from build123d import *

# Parameters (mm, degrees)
BOSS_EXTRUDE1_DEPTH   = 116
SKETCH5_R             = 16
CUT_EXTRUDE1_DEPTH    = 20
CUT_EXTRUDE2_REACH    = 6.51
SKETCH6_R             = 10
CUT_EXTRUDE4_REACH    = 17
SKETCH8_R             = 45
CUT_EXTRUDE5_DEPTH    = 106
FILLET3_R             = 25
SKETCH21_R            = 55
CUT_EXTRUDE7_DEPTH    = 5
M4X0_7_TAPPED_HOLE1_D = 3.3
FILLET4_R             = 0.8
CHAMFER1_SIZE         = 10
SKETCH25_W            = 64.356
SKETCH25_H            = 48.356
BOSS_EXTRUDE2_DEPTH   = 116
CUT_EXTRUDE8_DEPTH    = 106
FILLET6_R             = 10
FILLET7_R             = 10
FILLET8_R             = 10


with BuildPart() as part:
    # Sketch1 → Boss-Extrude1 (new body)
    with BuildSketch(Plane.XY):
        Polygon((0, 0), (-106, 0), (-121, 0), (-121, 155), (-106, 155), (-106, 16), (-24.51, 16), (-24.51, 107), (0, 107), align=None)
    extrude(amount=-BOSS_EXTRUDE1_DEPTH)

    # Sketch5 → Cut-Extrude1 (cut)
    with BuildSketch(Plane.ZY.offset(24.51)):
        with Locations((-58, 86)):
            Circle(SKETCH5_R)
    extrude(amount=-CUT_EXTRUDE1_DEPTH, mode=Mode.SUBTRACT)

    # Sketch6 → Cut-Extrude2 (cut, up to next)
    with BuildSketch(Plane.ZY.offset(4.51), mode=Mode.PRIVATE) as cut_extrude2_sk1:
        with Locations((-58, 86)):
            Circle(SKETCH6_R)
    cut_extrude2_tool1 = extrude(cut_extrude2_sk1.sketch, amount=-CUT_EXTRUDE2_REACH, mode=Mode.PRIVATE) & part.part
    add(cut_extrude2_tool1.solids().sort_by_distance((-4.51, 86, -58))[0], mode=Mode.SUBTRACT)

    # Sketch8 → Cut-Extrude4 (cut, up to next)
    with BuildSketch(Plane(origin=(-106, 0, 0), x_dir=(0, 0, -1), z_dir=(1, 0, 0)), mode=Mode.PRIVATE) as cut_extrude4_sk1:
        with Locations((58, 86)):
            Circle(SKETCH8_R)
    cut_extrude4_tool1 = extrude(cut_extrude4_sk1.sketch, amount=-CUT_EXTRUDE4_REACH, mode=Mode.PRIVATE) & part.part
    add(cut_extrude4_tool1.solids().sort_by_distance((-106, 86, -58))[0], mode=Mode.SUBTRACT)

    # Sketch10 → Cut-Extrude5 (cut)
    with BuildSketch(Plane(origin=(0, 0, 0), x_dir=(0, 0, -1), z_dir=(1, 0, 0))):
        with BuildLine():
            Line((0, 107), (0, 16))
            Line((0, 16), (23.561161531, 22.820336233))
            ThreePointArc((23.561161531, 22.820336233), (33.987858372, 30.015449722), (38, 42.031621521))
            Line((38, 42.031621521), (38, 87))
            ThreePointArc((38, 87), (43.857864376, 101.142135624), (58, 107))
            Line((58, 107), (0, 107))
        make_face()
        with BuildLine():
            Line((116, 107), (58, 107))
            ThreePointArc((58, 107), (72.142135624, 101.142135624), (78, 87))
            Line((78, 87), (78, 42.031621521))
            ThreePointArc((78, 42.031621521), (82.012141628, 30.015449722), (92.438838469, 22.820336233))
            Line((92.438838469, 22.820336233), (116, 16))
            Line((116, 16), (116, 107))
        make_face()
    extrude(amount=-CUT_EXTRUDE5_DEPTH, mode=Mode.SUBTRACT)

    # Fillet3
    fillet3_edges = [part.edges().sort_by_distance(p)[0] for p in [
        (-113.5, 155, 0),
        (-113.5, 155, -116),
    ]]
    fillet(fillet3_edges, radius=FILLET3_R)

    # Sketch21 → Cut-Extrude7 (cut)
    with BuildSketch(Plane.ZY.offset(121)):
        with Locations((-58, 86)):
            Circle(SKETCH21_R)
    extrude(amount=-CUT_EXTRUDE7_DEPTH, mode=Mode.SUBTRACT)

    # M4x0.7 Tapped Hole1 (through all)
    with Locations(Plane.ZY.offset(116)):
        with Locations((-103.10855484, 107.568919311), (-12.89144516, 107.568919311), (-12.89144516, 64.431080689), (-103.10855484, 64.431080689)):
            Hole(M4X0_7_TAPPED_HOLE1_D / 2)

    # Mirror1: part across plane


with BuildPart() as part_1:
    add(part.part)
    add(part.part.mirror(Plane(origin=(0, 107, -116), x_dir=(0, 0, 1), z_dir=(1, 0, 0))))

    # Fillet4
    fillet4_edges = [part_1.edges().sort_by_distance(p)[0] for p in [
        (4.51, 86, -74),
        (-4.51, 86, -74),
    ]]
    fillet(fillet4_edges, radius=FILLET4_R)

    # Chamfer1
    chamfer1_edges = [part_1.edges().sort_by_distance(p)[0] for p in [
        (-121, 0, -58),
        (121, 0, -58),
    ]]
    chamfer(chamfer1_edges, length=CHAMFER1_SIZE)

    # Sketch25 → Boss-Extrude2 (add)
    with BuildSketch(Plane.XY):
        with Locations((0, -24.178)):
            Rectangle(SKETCH25_W, SKETCH25_H)
    extrude(amount=-BOSS_EXTRUDE2_DEPTH)

    # Sketch27 → Cut-Extrude8 (cut)
    with BuildSketch(Plane(origin=(0, 0, -116), x_dir=(-1, 0, 0), z_dir=(0, 0, -1))):
        with BuildLine():
            Line((-21.05025, -43.356), (21.05025, -43.356))
            ThreePointArc((21.05025, -43.356), (25.383223578, -41.561223578), (27.178, -37.22825))
            Line((27.178, -37.22825), (27.178, 4.87225))
            ThreePointArc((27.178, 4.87225), (25.383223578, 9.205223578), (21.05025, 11))
            Line((21.05025, 11), (-21.05025, 11))
            ThreePointArc((-21.05025, 11), (-25.383223578, 9.205223578), (-27.178, 4.87225))
            Line((-27.178, 4.87225), (-27.178, -37.22825))
            ThreePointArc((-27.178, -37.22825), (-25.383223578, -41.561223578), (-21.05025, -43.356))
        make_face()
    extrude(amount=-CUT_EXTRUDE8_DEPTH, mode=Mode.SUBTRACT)

    # Fillet6
    fillet6_edges = [part_1.edges().sort_by_distance(p)[0] for p in [
        (-32.178, 0, -58),
        (32.178, 0, -58),
    ]]
    fillet(fillet6_edges, radius=FILLET6_R)

    # Fillet7
    fillet7_edges = [part_1.edges().sort_by_distance(p)[0] for p in [
        (-32.178, -48.356, -58),
        (32.178, -48.356, -58),
    ]]
    fillet(fillet7_edges, radius=FILLET7_R)

    # Fillet8
    fillet8_edges = [part_1.edges().sort_by_distance(p)[0] for p in [
        (106, 16, -58),
        (-106, 16, -58),
    ]]
    fillet(fillet8_edges, radius=FILLET8_R)


solid = part_1.part
The listing builds one solid part. Answer for the finished solid, in the listing's coordinates (mm). A direction names the side the tool comes from. Coordinates: 2 decimals unless noted, no trailing zeros. Write each loop counter-clockwise with the first axis right and the second up, starting at its lowest first coordinate (ties: lowest second). Pieces come first, ordered by that corner, then holes. Notation, with made-up numbers: (46, -3.75) -> (93, -3.75) arc R19 ccw to (93, 7.25) -> close; hole circle Ø8 at (-9, 87.25). An arc over 180 degrees is marked (long way). One line per question, with ' | ' between items.
1. For a pull along X with two mould halves and no side action, classify faces 5 (the flat face through (-106, 134, -57)), 6 (the flat face through (27.178, -16, -64)), 7 (the flat face through (116, 5, -57)), 8 (the flat face through (-1, 15, 0)) as released by +X, released by -X, zero draft, split by the parting line, or undercut.
Verdict:
face 5: undercut | face 6: undercut | face 7: released by +X | face 8: zero draft
2. Section C-C (x = 90) is taken. Determine the outline of the cut face in (y, z), and give its area (3 significant figures).
Verdict:
outline: (0, -116) -> (16, -116) -> (16, 0) -> (0, 0) -> close | area: 1,860 mm^2
3. Straight lines are drawn through the part: line 1 (Y direction, x = -10.5, z = -58); line 2 (X direction, y = -17, z = -29.5); line 3 (X direction, y = 136, z = -65). For each, find the intervals that lie inside material, in ascending order.
Verdict:
line 1: y = -48.36 to -43.36, 11 to 70, 102 to 107 | line 2: x = -32.18 to -27.18, 27.18 to 32.18 | line 3: x = -116 to -106, 106 to 116
4. Which of the six approach directions +Z, -Z, +X, -X, +Y, -Y give full straight-line access (tool end or side, diameter ignored) to faces 1 (the cylindrical face through (-118.535, 64.935, -7.194)), 2 (the cylindrical face through (-0.3, 29.9, -33.9)), 3 (the flat face through (77, 0, -57)), 4 (the cylindrical face through (25.34, 9.25, -63.74))?
Verdict:
face 1: -X | face 2: +Z, +Y | face 3: +Z, -Z, +X, -Y | face 4: -Z
5. Given pin 1 Ø5.5 at (y, z) = (107.57, -12.89) entering from +X; pin 2 Ø1 at (x, z) = (47, -93.5) entering from -Y; pin 3 Ø3 at (y, z) = (92, -73.5) entering from +X, each flat-ended and moving along its own axis, determine where each tip first touches the part or whether it passes through.
Verdict:
pin 1: stops at x = 116 | pin 2: stops at y = 0 | pin 3: stops at x = 24.51
6. Section A-A (y = 49) is taken. Determine the outline of the cut face in (x, z).
Verdict:
outline: (-121, -116) -> (-106, -116) -> (-106, -83.61) -> (-116, -83.61) -> (-116, -98.69) -> (-121, -98.69) -> close; (-121, -17.31) -> (-116, -17.31) -> (-116, -32.39) -> (-106, -32.39) -> (-106, 0) -> (-121, 0) -> close; (-24.51, -78) -> (24.51, -78) -> (24.51, -38) -> (-24.51, -38) -> close; (106, -116) -> (121, -116) -> (121, -98.69) -> (116, -98.69) -> (116, -83.61) -> (106, -83.61) -> close; (106, -32.39) -> (116, -32.39) -> (116, -17.31) -> (121, -17.31) -> (121, 0) -> (106, 0) -> close
7. Section B-B (z = -58) is taken. State how many separate pieces and enclosed holes the cut face has, and give its area (3 significant figures).
Verdict:
separate pieces: 4 | enclosed holes: 1 | area: 8,280 mm^2
